from build123d import *

# Parameters (mm, degrees)
SKETCH_1_W          = 41
SKETCH_1_H          = 34
SKETCH_1_W_2        = 37
SKETCH_1_H_2        = 30
EXTRUDE_1_DEPTH     = 34
SKETCH_2_W          = 15
SKETCH_2_H          = 3
EXTRUDE_2_DEPTH     = 10
SKETCH_3_R          = 2.008063055
CUT_EXTRUDE_1_DEPTH = 10
SKETCH_4_W          = 25
SKETCH_4_H          = 30
CUT_EXTRUDE_2_DEPTH = 60


with BuildPart() as part:
    # 草圖1 → 填料-伸長1 (new body)
    with BuildSketch(Plane.XY):
        Rectangle(SKETCH_1_W, SKETCH_1_H)
        Rectangle(SKETCH_1_W_2, SKETCH_1_H_2, mode=Mode.SUBTRACT)
    extrude(amount=EXTRUDE_1_DEPTH)

    # 草圖2 → 填料-伸長2 (add)
    with BuildSketch(Plane(origin=(0, 17, 0), x_dir=(1, 0, 0), z_dir=(0, 1, 0))):
        with Locations((0, -1.5)):
            Rectangle(SKETCH_2_W, SKETCH_2_H)
    extrude_2 = extrude(amount=EXTRUDE_2_DEPTH)

    # 草圖3 → 除料-伸長1 (cut)
    with BuildSketch(Plane.XY.offset(3)):
        with Locations((0, 22)):
            Circle(SKETCH_3_R)
    cut_extrude_1 = extrude(amount=-CUT_EXTRUDE_1_DEPTH, mode=Mode.SUBTRACT)

    # 鏡射1: 填料-伸長2, 除料-伸長1 across plane
    add(extrude_2.mirror(Plane.ZX))
    add(cut_extrude_1.mirror(Plane.ZX), mode=Mode.SUBTRACT)

    # 草圖4 → 除料-伸長2 (cut)
    with BuildSketch(Plane.ZY.offset(20.5)):
        with Locations((12.5, 0)):
            Rectangle(SKETCH_4_W, SKETCH_4_H)
    extrude(amount=-CUT_EXTRUDE_2_DEPTH, mode=Mode.SUBTRACT)


solid = part.part
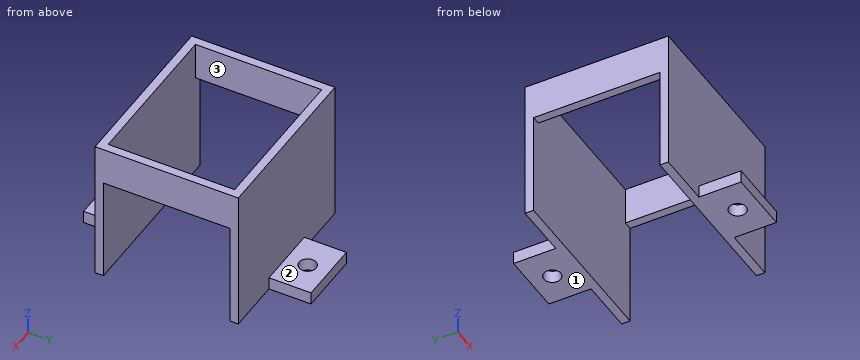
Work out the finished part from the listing and answer in its coordinate system (mm). Face numbers are marked on the shaded views. A direction names the side the tool comes from. Round coordinates to 2 decimals unless told otherwise and drop trailing zeros. Write each loop counter-clockwise with the first axis right and the second up, starting at its lowest first coordinate (ties: lowest second). Pieces come first, ordered by that corner, then holes.
1) Straight lines are drawn through the part: line 1 (Y direction, x = 0, z = 1.2); line 2 (Y direction, x = 14, z = 20.5); line 3 (X direction, y = -22, z = 2). For each, find the intervals that lie inside material, in ascending order.
2) A cutting plane is placed at A-A (z = 2). Give the vertices of the cut face in (x, y).
3) A cutting plane is placed at B-B (x = 15). Give the vertices of the cut face in (y, z).
4) Given pin 1 Ø2.5 at (y, z) = (22.5, 1) entering from -X; pin 2 Ø11 at (x, y) = (-0.5, 23) entering from +Z; pin 3 Ø2 at (x, y) = (19.5, -1.5) entering from -Z, each flat-ended and moving along its own axis, determine where each tip first touches the part or whether it passes through.
5) A tool of negligible diameter and unlimited length cuts with its end or side. For the marked faces 1, 2 and 3, from which of +Z, -Z, +X, -X, +Y, -Y can it reach the whole face along a straight path? Write none if from no direction.
6) A cutting plane is placed at C-C (y = -22). Give the vertices of the cut face in (x, z), plus the area to 3 significant figures.
7) A cutting plane is placed at D-D (x = 0). Give the vertices of the cut face in (y, z).
Completed:
1. line 1: y = -27 to -24.01, -19.99 to -15, 15 to 19.99, 24.01 to 27
1. line 2: y = -17 to -15, 15 to 17
1. line 3: x = -7.5 to -2.01, 2.01 to 7.5
2. outline: (-20.5, -17) - (-7.5, -17) - (-7.5, -27) - (7.5, -27) - (7.5, -17) - (20.5, -17) - (20.5, -15) - (-20.5, -15) - close; (-20.5, 15) - (20.5, 15) - (20.5, 17) - (7.5, 17) - (7.5, 27) - (-7.5, 27) - (-7.5, 17) - (-20.5, 17) - close; hole circle Ø4.02 at (0, -22); hole circle Ø4.02 at (0, 22)
3. outline: (-17, 0) - (-15, 0) - (-15, 34) - (-17, 34) - close; (15, 0) - (17, 0) - (17, 34) - (15, 34) - close
4. pin 1: stops at x = -7.5
4. pin 2: stops at z = 3
4. pin 3: stops at z = 25
5. face 1: -Z, +X, -X, +Y, -Y
5. face 2: +Z, +X, -X, +Y
5. face 3: +Z, -Z
6. outline: (-7.5, 0) - (-2.01, 0) - (-2.01, 3) - (-7.5, 3) - close; (2.01, 0) - (7.5, 0) - (7.5, 3) - (2.01, 3) - close
6. area: 33.0 mm2
7. outline: (-27, 0) - (-24.01, 0) - (-24.01, 3) - (-27, 3) - close; (-19.99, 0) - (-15, 0) - (-15, 34) - (-17, 34) - (-17, 3) - (-19.99, 3) - close; (15, 0) - (19.99, 0) - (19.99, 3) - (17, 3) - (17, 34) - (15, 34) - close; (24.01, 0) - (27, 0) - (27, 3) - (24.01, 3) - close
